```python
from build123d import *

# Parameters (mm, degrees)
SKETCH2_R            = 22.1488
BOSS_EXTRUDE4_DEPTH  = 66.0908
SKETCH4_R            = 8.6995
BOSS_EXTRUDE5_DEPTH  = 5.0038
SKETCH9_R            = 2.5019
BOSS_EXTRUDE6_DEPTH  = 7.7978
SKETCH10_R           = 8.7503
BOSS_EXTRUDE7_DEPTH  = 6.7056
SKETCH11_R           = 2.5019
BOSS_EXTRUDE8_DEPTH  = 2.413
SKETCH12_R           = 23.8125
BOSS_EXTRUDE9_DEPTH  = 34.0106
SKETCH13_R           = 2.0955
CUT_EXTRUDE1_DEPTH   = 3.175
CUT_EXTRUDE2_DEPTH   = 3.175
SKETCH15_R           = 20.958175
SKETCH15_R_2         = 8.7503
CUT_EXTRUDE3_DEPTH   = 3.175
SKETCH16_R           = 7.1628
SKETCH16_R_2         = 2.5019
CUT_EXTRUDE4_DEPTH   = 2.54
BOSS_EXTRUDE12_DEPTH = 3.175
BOSS_EXTRUDE13_DEPTH = 3.175
SKETCH20_R           = 1.5875
CUT_EXTRUDE5_DEPTH   = 3.175


with BuildPart() as part:
    # Sketch2 → Boss-Extrude4 (new body)
    with BuildSketch(Plane(origin=(0, 0, 0), x_dir=(1, 0, 0), z_dir=(0, 1, 0))):
        Circle(SKETCH2_R)
    extrude(amount=BOSS_EXTRUDE4_DEPTH)

    # Sketch4 → Boss-Extrude5 (add)
    with BuildSketch(Plane(origin=(0, 66.0908, 0), x_dir=(1, 0, 0), z_dir=(0, 1, 0))):
        Circle(SKETCH4_R)
    extrude(amount=BOSS_EXTRUDE5_DEPTH)

    # Sketch9 → Boss-Extrude6 (add)
    with BuildSketch(Plane(origin=(0, 71.0946, 0), x_dir=(1, 0, 0), z_dir=(0, 1, 0))):
        Circle(SKETCH9_R)
    extrude(amount=BOSS_EXTRUDE6_DEPTH)

    # Sketch10 → Boss-Extrude7 (add)
    with BuildSketch(Plane.XZ):
        Circle(SKETCH10_R)
    extrude(amount=BOSS_EXTRUDE7_DEPTH)

    # Sketch11 → Boss-Extrude8 (add)
    with BuildSketch(Plane.XZ.offset(6.7056)):
        Circle(SKETCH11_R)
    extrude(amount=BOSS_EXTRUDE8_DEPTH)

    # Sketch12 → Boss-Extrude9 (add)
    with BuildSketch(Plane(origin=(0, 53.1114, 0), x_dir=(-1, 0, 0), z_dir=(0, -1, 0))):
        Circle(SKETCH12_R)
    extrude(amount=BOSS_EXTRUDE9_DEPTH)

    # Sketch13 → Cut-Extrude1 (cut)
    with BuildSketch(Plane(origin=(0, 66.0908, 0), x_dir=(1, 0, 0), z_dir=(0, 1, 0))):
        with Locations((-14.5034, 0)):
            Circle(SKETCH13_R)
        with Locations((14.5034, 0)):
            Circle(SKETCH13_R)
    extrude(amount=-CUT_EXTRUDE1_DEPTH, mode=Mode.SUBTRACT)

    # Sketch14 → Cut-Extrude2 (cut)
    with BuildSketch(Plane(origin=(0, 66.0908, 0), x_dir=(1, 0, 0), z_dir=(0, 1, 0))):
        with BuildLine():
            Line((-14.070005184, -6.560951168), (-17.033311719, -7.942763698))
            ThreePointArc((-17.033311719, -7.942763698), (-13.856523006, -12.697163994), (-9.397090019, -16.276237356))
            Line((-9.397090019, -16.276237356), (-7.76226652, -13.444639995))
            ThreePointArc((-7.76226652, -13.444639995), (-11.445886375, -10.4882225), (-14.070005184, -6.560951168))
        make_face()
        with BuildLine():
            ThreePointArc((-10.080336815, 15.862156631), (-14.123267338, 12.399779151), (-17.033311719, 7.942763698))
            Line((-17.033311719, 7.942763698), (-14.070005184, 6.560951168))
            ThreePointArc((-14.070005184, 6.560951168), (-11.711998853, 10.190201616), (-8.44372295, 13.027458265))
            Line((-8.44372295, 13.027458265), (-10.080336815, 15.862156631))
        make_face()
        with BuildLine():
            ThreePointArc((17.033311719, 7.942763698), (13.856523006, 12.697163994), (9.397090019, 16.276237356))
            Line((9.397090019, 16.276237356), (7.76226652, 13.444639995))
            ThreePointArc((7.76226652, 13.444639995), (11.445886375, 10.4882225), (14.070005184, 6.560951168))
            Line((14.070005184, 6.560951168), (17.033311719, 7.942763698))
        make_face()
        with BuildLine():
            Line((9.385927189, -12.365900571), (11.031460095, -15.21604717))
            ThreePointArc((11.031460095, -15.21604717), (14.495965555, -11.961947414), (17.033311719, -7.942763698))
            Line((17.033311719, -7.942763698), (14.070005184, -6.560951168))
            ThreePointArc((14.070005184, -6.560951168), (12.081785889, -9.748926908), (9.385927189, -12.365900571))
        make_face()
    extrude(amount=-CUT_EXTRUDE2_DEPTH, mode=Mode.SUBTRACT)

    # Sketch15 → Cut-Extrude3 (cut)
    with BuildSketch(Plane.XZ):
        Circle(SKETCH15_R)
        Circle(SKETCH15_R_2, mode=Mode.SUBTRACT)
    extrude(amount=-CUT_EXTRUDE3_DEPTH, mode=Mode.SUBTRACT)

    # Sketch16 → Cut-Extrude4 (cut)
    with BuildSketch(Plane.XZ.offset(6.7056)):
        Circle(SKETCH16_R)
        Circle(SKETCH16_R_2, mode=Mode.SUBTRACT)
    extrude(amount=-CUT_EXTRUDE4_DEPTH, mode=Mode.SUBTRACT)

    # Sketch18 → Boss-Extrude12 (add)
    with BuildSketch(Plane.XZ):
        with BuildLine():
            ThreePointArc((20.865163654, 0), (20.780212376, 1.88091146), (20.52605029, 3.746506881))
            Line((20.52605029, 3.746506881), (17.399, 3.746506881))
            Line((17.399, 3.746506881), (17.399, -2.603493119))
            Line((17.399, -2.603493119), (20.702098393, -2.603493119))
            ThreePointArc((20.702098393, -2.603493119), (20.824357436, -1.304297387), (20.865163654, 0))
        make_face()
    extrude(amount=-BOSS_EXTRUDE12_DEPTH)

    # Sketch19 → Boss-Extrude13 (add)
    with BuildSketch(Plane(origin=(0, 0, 0), x_dir=(-1, 0, 0), z_dir=(0, -1, 0))):
        with BuildLine():
            Line((20.716285244, -3.175), (17.399, -3.175))
            Line((17.399, -3.175), (17.399, 3.175))
            Line((17.399, 3.175), (20.716285244, 3.175))
            ThreePointArc((20.716285244, 3.175), (20.958175, 0), (20.716285244, -3.175))
        make_face()
    extrude(amount=-BOSS_EXTRUDE13_DEPTH)

    # Sketch20 → Cut-Extrude5 (cut)
    with BuildSketch(Plane(origin=(0, 3.175, 0), x_dir=(-1, 0, 0), z_dir=(0, -1, 0))):
        with Locations((-15.1765, 6.730993119)):
            Circle(SKETCH20_R)
    extrude(amount=-CUT_EXTRUDE5_DEPTH, mode=Mode.SUBTRACT)


solid = part.part
```
Source: CAD feature listing. Evaluate the final solid. Frame: model axes, mm. A direction names the side the tool comes from. Coordinates: 2 decimals unless noted, no trailing zeros. Loops run counter-clockwise (first coordinate to the right, second up) from the corner with the lowest first, then second, coordinate; pieces in that order, holes last. Notation, with made-up numbers: M 73,-22 L 78,-22 A26 cw 78,-6 Z; hole C -32.5,50.5 d9. An arc over 180 degrees is marked long. Put each result on its own line as item: value. Start each with the question number.
1) Pull-direction query (X, two-part tool) for faces 4 (the face through (-17.399, 2, 0)), 5 (the face through (2, 71.095, 2)), 6 (the face through (-1.89, 68.56, 8.49)); classes: pulls with the +X half, pulls with the -X half, needs draft (parallel to the pull), parting line crosses it, or undercut.
2) Reachability of faces 1 (the face through (19, 0, 1)), 2 (the face through (10.197, 64.526, 13.771)), 3 (the face through (-16, 19.101, 16)) from +Z, -Z, +X, -X, +Y, -Y: full face, straight path, thin tool, end or side. Return the list, or none.
3) Cut plane C-C on y = 40.5. Return the cut outline in (x, z) (1 decimal), then the cut area to 3 significant figures.
4) Contact query for flat-ended pins moving along their axis: pin 1 Ø12 at (x, y) = (8, 56) entering from +Z; pin 2 Ø1 at (x, z) = (12.5, 7.5) entering from +Y; pin 3 Ø6.5 at (x, z) = (14.5, 0) entering from -Y. Output: stop coordinate, or through.
5) Cut plane B-B on z = -11.5. Return the cut outline in (x, y) (1 decimal), then the cut area to 3 significant figures.
6) Cut plane A-A on y = 1. Return the cut outline in (x, z) (1 decimal), then the cut area to 3 significant figures.
7) Ray query, L1, parallel to Z at x = 0, y = -5.3; L2, parallel to X at y = 65.4, z = 0; L3, parallel to Y at x = 5, z = 3. Return the intervals inside material, ascending. Write a range as from..to.
8) Cut plane D-D on y = 69. Return the cut outline in (x, z).
The answers:
1. face 4: undercut
1. face 5: needs draft
1. face 6: parting line crosses it
2. face 1: +Z, -Z, +X, -Y
2. face 2: +Y
2. face 3: -Y
3. outline: C 0,0 d47.6
3. area: 1,780 mm²
4. pin 1: stops at z = 23.65
4. pin 2: stops at y = 66.09
4. pin 3: stops at y = 0
5. outline: M -20.9,19.1 L -18.9,19.1 L -18.9,0 L -17.5,0 L -17.5,3.2 L 17.5,3.2 L 17.5,0 L 18.9,0 L 18.9,19.1 L 20.9,19.1 L 20.9,53.1 L 18.9,53.1 L 18.9,66.1 L 14.9,66.1 L 14.9,62.9 L 10.4,62.9 L 10.4,66.1 L -10.4,66.1 L -10.4,62.9 L -14.9,62.9 L -14.9,66.1 L -18.9,66.1 L -18.9,53.1 L -20.9,53.1 Z
5. area: 2,490 mm²
6. outline: C 0,0 d44.3; C 0,0 d17.5; M 17.4,-2.6 L 20.7,-2.6 A20.9 ccw 20.5,3.7 L 17.4,3.7 Z; hole M -20.7,-3.2 A21 ccw long -20.7,3.2 L -17.4,3.2 L -17.4,-3.2 Z
6. area: 445 mm²
7. L1: z = -8.75..-7.16, -2.5..2.5, 7.16..8.75
7. L2: x = -22.15..-16.6, -12.41..12.41, 16.6..22.15
7. L3: y = -4.17..71.09
8. outline: C 0,0 d17.4
